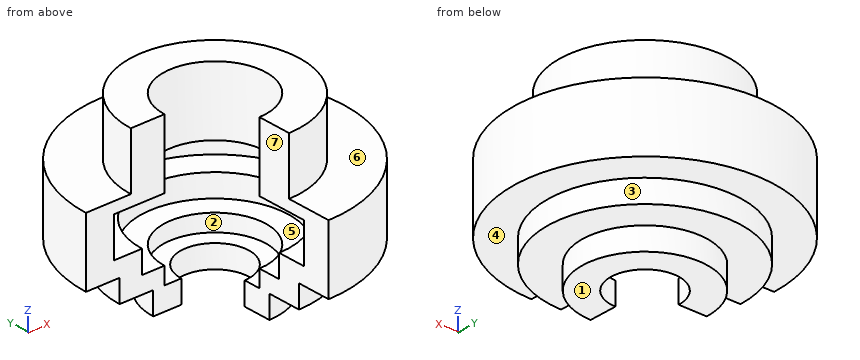
from build123d import *

# Parameters (mm, degrees)
REVOLVE1_ANGLE = 270


with BuildPart() as part:
    # Sketch1 → Revolve1 (revolve)
    with BuildSketch(Plane(origin=(0, 0, 0), x_dir=(1, 0, 0), z_dir=(0, 1, 0))):
        Polygon((-60, 150), (-110, 150), (-110, 110), (-170, 110), (-170, 70), (-230, 70), (-230, -50), (-150, -50), (-150, -150), (-90, -150), (-90, -30), (-180, -30), (-180, 40), (-130, 40), (-130, 80), (-90, 80), (-90, 110), (-60, 110), align=None)
    revolve(axis=Axis((0, 0, 150), (0, 0, -1)), revolution_arc=REVOLVE1_ANGLE)


solid = part.part
Build history of the part. All positions in model axes, mm. Face numbers are marked on the shaded views. A direction names the side the tool comes from. Coordinates: 2 decimals unless noted, no trailing zeros. Write each loop counter-clockwise with the first axis right and the second up, starting at its lowest first coordinate (ties: lowest second). Pieces come first, ordered by that corner, then holes.
(1) Pin check, flat tips, straight feed: pin 1 Ø8 at (y, z) = (-100, -18.5) entering from +X; pin 2 Ø10 at (x, y) = (78, 103.5) entering from -Z; pin 3 Ø1 at (x, z) = (-35, 71) entering from +Y. Stop position of each tip, or through.
(2) Cut at D-D on z = -18. List the corners of the cut face in (x, y), and give its area (3 significant figures).
(3) Cut at C-C on x = 104. List the corners of the cut face in (y, z), and give its area (3 significant figures).
(4) Drill centre lines: line 1 (Z direction, x = -166, y = 2.5); line 2 (Z direction, x = 122, y = 126); line 3 (Y direction, x = -120, z = 103). Where is each one in solid material? Low to high.
(5) Cut at B-B on y = -9. List the corners of the cut face in (x, z), and give its area (3 significant figures).
(6) Cut at A-A on x = -28. List the corners of the cut face in (y, z), and give its area (3 significant figures).
(7) Mould opens along Y. For the marked faces 1, 2 and 3 say: pulls with the +Y half, pulls with the -Y half, needs draft (parallel to the pull), parting line crosses it, or undercut.
(8) 3-axis set-ups, long thin cutter, end or side, ignore diameter. For the marked faces 4, 5, 6 and 7: which of +Z, -Z, +X, -X, +Y, -Y reach the whole face in a straight line?
Working result:
1. pin 1: stops at x = 209.01
1. pin 2: stops at z = -110
1. pin 3: stops at y = 145.98
2. outline: (-230, 0) - (-180, 0) arc R180 cw (long way) to (0, -180) - (0, -230) arc R230 ccw (long way) to start
2. area: 48,300 mm2
3. outline: (-205.14, -70) - (-134.48, -70) - (-134.48, -110) - (-35.83, -110) - (-35.83, -150) - (35.83, -150) - (35.83, -110) - (134.48, -110) - (134.48, -70) - (205.14, -70) - (205.14, 50) - (108.09, 50) - (108.09, 150) - (-108.09, 150) - (-108.09, 50) - (-205.14, 50) - close; hole (-146.91, -40) - (-78, -40) - (-78, -80) - (78, -80) - (78, -40) - (146.91, -40) - (146.91, 30) - (-146.91, 30) - close
3. area: 57,700 mm2
4. line 1: z = -110 to -40, 30 to 50
4. line 2: z = -70 to -40, 30 to 50
4. line 3: y = 0 to 90
5. outline: (59.32, -150) - (109.63, -150) - (109.63, -110) - (169.76, -110) - (169.76, -70) - (229.82, -70) - (229.82, 50) - (149.73, 50) - (149.73, 150) - (89.55, 150) - (89.55, 30) - (179.77, 30) - (179.77, -40) - (129.69, -40) - (129.69, -80) - (89.55, -80) - (89.55, -110) - (59.32, -110) - close
5. area: 20,200 mm2
6. outline: (53.07, -150) - (106.38, -150) - (106.38, -110) - (167.68, -110) - (167.68, -70) - (228.29, -70) - (228.29, 50) - (147.36, 50) - (147.36, 150) - (85.53, 150) - (85.53, 30) - (177.81, 30) - (177.81, -40) - (126.95, -40) - (126.95, -80) - (85.53, -80) - (85.53, -110) - (53.07, -110) - close
6. area: 20,600 mm2
7. face 1: needs draft
7. face 2: undercut
7. face 3: parting line crosses it
8. face 4: -Z
8. face 5: none
8. face 6: +Z
8. face 7: +Z, -Z, -X, -Y
